```python
from build123d import *

# Parameters (mm, degrees)
SKETCH1_W                     = 118.11
SKETCH1_H                     = 118.11
BOSS_EXTRUDE1_DEPTH           = 15
CBORE_FOR_M6_SHCS1_AT_2_COUNT = 2
CBORE_FOR_M6_SHCS1_AT_2_PITCH = 75
CBORE_FOR_M6_SHCS1_AT_3_COUNT = 2
CBORE_FOR_M6_SHCS1_AT_3_PITCH = 106.066017178
CBORE_FOR_M6_SHCS1_AT_4_COUNT = 2
CBORE_FOR_M6_SHCS1_AT_4_PITCH = 75
M6X1_0_TAPPED_HOLE1_D         = 5
M6X1_0_TAPPED_HOLE1_DEPTH     = 10
M6X1_0_TAPPED_HOLE1_TIP       = 1.502151548


with BuildPart() as part:
    # Sketch1 → Boss-Extrude1 (new body)
    with BuildSketch(Plane(origin=(0, 0, 0), x_dir=(1, 0, 0), z_dir=(0, 1, 0))):
        Rectangle(SKETCH1_W, SKETCH1_H)
    extrude(amount=-BOSS_EXTRUDE1_DEPTH)

    # Sketch5 → CBORE for M6 SHCS1 (revolve, cut)
    with BuildSketch(Plane(origin=(-37.5, 0, 37.5), x_dir=(0, 0, 1), z_dir=(1, 0, 0))):
        Polygon((0, 0), (0, 16.982840043), (3.3, 15), (3.3, 7), (5.5, 7), (5.5, 0.025), (5.525, 0), align=None)
    cbore_for_m6_shcs1 = revolve(axis=Axis((-37.5, 6.35, 37.5), (0, -1, 0)), mode=Mode.SUBTRACT)

    # CBORE for M6 SHCS1 at 2: CBORE for M6 SHCS1 ×2
    with Locations(*[(i * CBORE_FOR_M6_SHCS1_AT_2_PITCH, 0, 0) for i in range(1, CBORE_FOR_M6_SHCS1_AT_2_COUNT)]):
        add(cbore_for_m6_shcs1, mode=Mode.SUBTRACT)

    # CBORE for M6 SHCS1 at 3: CBORE for M6 SHCS1 ×2
    with Locations(*[Vector(0.707106781, 0, -0.707106781) * (i * CBORE_FOR_M6_SHCS1_AT_3_PITCH) for i in range(1, CBORE_FOR_M6_SHCS1_AT_3_COUNT)]):
        add(cbore_for_m6_shcs1, mode=Mode.SUBTRACT)

    # CBORE for M6 SHCS1 at 4: CBORE for M6 SHCS1 ×2
    with Locations(*[(0, 0, -i * CBORE_FOR_M6_SHCS1_AT_4_PITCH) for i in range(1, CBORE_FOR_M6_SHCS1_AT_4_COUNT)]):
        add(cbore_for_m6_shcs1, mode=Mode.SUBTRACT)

    # M6x1.0 Tapped Hole1
    with Locations(Plane(origin=(0, 0, 0), x_dir=(1, 0, 0), z_dir=(0, 1, 0))):
        with Locations((-50.8, -50.8), (-50.8, 50.8), (50.8, 50.8), (50.8, -50.8)):
            Hole(M6X1_0_TAPPED_HOLE1_D / 2, depth=M6X1_0_TAPPED_HOLE1_DEPTH)
            with Locations((0, 0, -(M6X1_0_TAPPED_HOLE1_DEPTH + M6X1_0_TAPPED_HOLE1_TIP / 2))):  # 118° drill point
                Cone(0, M6X1_0_TAPPED_HOLE1_D / 2, M6X1_0_TAPPED_HOLE1_TIP, mode=Mode.SUBTRACT)


solid = part.part
```
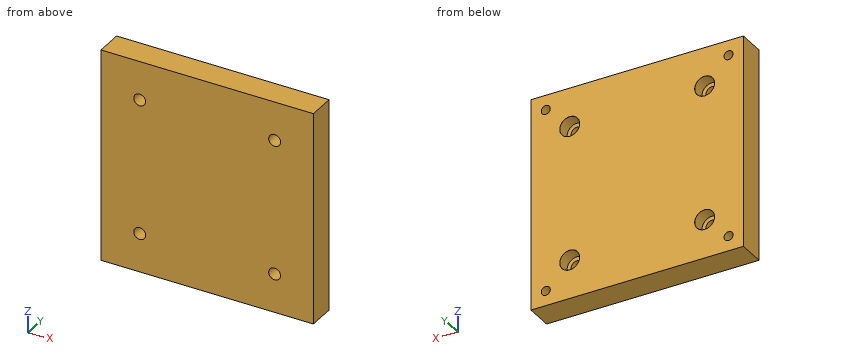
Input: part model. Units: mm. Frame: model coordinates. Give positions to 0.01 mm unless a question says otherwise; leave off trailing zeros. Loops run counter-clockwise (first coordinate to the right, second up) from the corner with the lowest first, then second, coordinate; pieces in that order, holes last.
1) Section query B-B on y = -3.5. Count the separate pieces of the cut face and the enclosed holes in it, and give its area (3 significant figures).
A:
separate pieces: 1
enclosed holes: 8
area: 13,500 mm2
2) Contact query for flat-ended pins moving along their axis: pin 1 (7.5 mm diameter, centred on x = 37.5, z = -37.5, fed in from +Y); pin 2 (6 mm diameter, centred on x = -37.5, z = -37.5, fed in from +Y). Output: stop coordinate, or through.
A:
pin 1: stops at y = -7
pin 2: passes through
3) Section query A-A on x = 37.5. Return the cut outline in (y, z) (3 decimals), and give its area (3 significant figures).
A:
outline: (-15, -59.055) - (0, -59.055) - (0, -43.025) - (-0.025, -43) - (-7, -43) - (-7, -40.8) - (-15, -40.8) - close; (-15, -34.2) - (-7, -34.2) - (-7, -32) - (-0.025, -32) - (0, -31.975) - (0, 31.975) - (-0.025, 32) - (-7, 32) - (-7, 34.2) - (-15, 34.2) - close; (-15, 40.8) - (-7, 40.8) - (-7, 43) - (-0.025, 43) - (0, 43.025) - (0, 59.055) - (-15, 59.055) - close
area: 1,510 mm2
4) Line query: L1, parallel to Z at x = 50.8, y = -7.25 (3 decimals); L2, parallel to X at y = -5.5, z = -37.5 (3 decimals); L3, parallel to X at y = -12, z = -37.5 (3 decimals). Output: solid intervals per line, ascending.
A:
L1: z = -59.055 to -53.3, -48.3 to 48.3, 53.3 to 59.055
L2: x = -59.055 to -43, -32 to 32, 43 to 59.055
L3: x = -59.055 to -40.8, -34.2 to 34.2, 40.8 to 59.055
